Model file for the job. Use its own axes, mm. A direction names the side the tool comes from. Give positions to 0.01 mm unless a question says otherwise; leave off trailing zeros. Loops run counter-clockwise (first coordinate to the right, second up) from the corner with the lowest first, then second, coordinate; pieces in that order, holes last. Notation, with made-up numbers: M 33,-2.5 L 80,-2.5 A25 cw 80,35.5 Z; hole C 30.5,58.5 d9. An arc over 180 degrees is marked long. Answer in a Markdown table with one row per item.
```python
from build123d import *

# Parameters (mm, degrees)
F3_DEPTH = 1.8
F4_R     = 0.75
F5_SIZE  = 0.5


with BuildPart() as f1:
    # F0 (on Front) → F1 (revolve)
    with BuildSketch(Plane.XZ):
        Polygon((0, 27.9), (0, 0), (1.5, 0), (1.5, 25), (2.7, 25), (2.7, 27.9), align=None)
    revolve(axis=Axis((0, 0, 13.95), (0, 0, 1)))

    # F2 (on face) → F3 (cut)
    with BuildSketch(Plane.XY.offset(27.9)):
        Polygon((0.750555, 1.3), (-0.750555, 1.3), (-1.501111, 0), (-0.750555, -1.3), (0.750555, -1.3), (1.501111, 0), align=None)
    extrude(amount=-F3_DEPTH, mode=Mode.SUBTRACT)

    # F4
    f4_edges = [f1.edges().sort_by_distance(p)[0] for p in [
        (-2.7, 0, 27.9),
    ]]
    fillet(f4_edges, radius=F4_R)

    # F5
    f5_edges = [f1.edges().sort_by_distance(p)[0] for p in [
        (-1.5, 0, 0),
    ]]
    chamfer(f5_edges, length=F5_SIZE)


solid = f1.part
```
(1) Which spindle directions (+Z, -Z, +X, -X, +Y, -Y) get a long thin tool onto all of the face, cutting with end or side? Do faces 4 (the cylindrical face through (-0.585, -2.636, 26.09)), 5 (the flat face through (-1.12, 0.66, 27.01)), 6 (the flat face through (-1.2, -1.2, 25)). Say none if no direction does.
Established:
| item | result |
|---|---|
| face 4 | +Z, -Z |
| face 5 | +Z |
| face 6 | -Z |
(2) Wall check: L1, parallel to Y at x = 0.05, z = 6.5; L2, parallel to X at y = -0.2, z = 8.5; L3, parallel to Z at x = -1.35, y = -1.9. Give the ranges that are in metal, low to high.
Established:
| item | result |
|---|---|
| L1 | y = -1.5 to 1.5 |
| L2 | x = -1.49 to 1.49 |
| L3 | z = 25 to 27.8 |
(3) Saw through at C-C, the plane z = 15.25. Give the cut face in (x, y), and give its area (3 significant figures).
Established:
| item | result |
|---|---|
| outline | C 0,0 d3 |
| area | 7.07 mm2 |
(4) Mould opens along Y. For faces 1 (the flat face through (1.13, 0.64, 27.01)), 2 (the cylindrical face through (-1.5, 0.07, 12.92)), 3 (the flat face through (0, 0, 0)) say: pulls with the +Y half, pulls with the -Y half, needs draft (parallel to the pull), parting line crosses it, or undercut.
Established:
| item | result |
|---|---|
| face 1 | undercut |
| face 2 | parting line crosses it |
| face 3 | needs draft |
(5) Flat gauge pins, fed straight in: P1, Ø1, axis at y = 0.5, z = 22, coming from the +X side; P2, Ø1.5, axis at x = 2, y = 1.5, coming from the -Z side; P3, Ø0.5, axis at x = -0.5, z = 27, coming from the -Y side. Where does each tip first touch, or does it go through?
Established:
| item | result |
|---|---|
| P1 | stops at x = 1.5 |
| P2 | stops at z = 25 |
| P3 | stops at y = -2.69 |
(6) Saw through at B-B, the plane z = 25.5. Give the cut face in (x, y), and give its area (3 significant figures).
Established:
| item | result |
|---|---|
| outline | C 0,0 d5.4 |
| area | 22.9 mm2 |
(7) Saw through at A-A, the plane x = 0. Give the cut face in (y, z), and give its area (3 significant figures).
Established:
| item | result |
|---|---|
| outline | M -2.7,25 L -1.5,25 L -1.5,0.5 L -1,0 L 1,0 L 1.5,0.5 L 1.5,25 L 2.7,25 L 2.7,27.15 A0.75 ccw 1.95,27.9 L 1.3,27.9 L 1.3,26.1 L -1.3,26.1 L -1.3,27.9 L -1.95,27.9 A0.75 ccw -2.7,27.15 Z |
| area | 85.5 mm2 |
